Design review of the part built by this model. Coordinates are the model's own, in mm. A direction names the side the tool comes from. Round coordinates to 2 decimals unless told otherwise and drop trailing zeros. Order: outer loops, then holes, each group sorted by start corner. A loop starts at its lowest first (then second) coordinate and runs counter-clockwise, first axis right, second up.
from build123d import *

# Parameters (mm, degrees)
F1_DEPTH = 6.35
F2_W     = 6.35
F2_H     = 12.7
F3_DEPTH = 12.7


with BuildPart() as f1:
    # F0 (on Right) → F1 (new body, symmetric)
    with BuildSketch(Plane.YZ):
        Polygon((2.713958, 14.533968), (23.782384, 14.533968), (11.706621, 68.364052), (-39.854848, 68.364052), (-39.854848, 74.714052), (-52.554848, 74.714052), (-52.554848, 55.664052), (-1.754848, 55.664052), align=None)
    extrude(amount=F1_DEPTH, both=True)

    # F2 (on face) → F3 (join)
    with BuildSketch(Plane(origin=(0, 0, 14.533968), x_dir=(1, 0, 0), z_dir=(0, 0, -1))):
        with Locations((0, -14.143958)):
            Rectangle(F2_W, F2_H)
    extrude(amount=F3_DEPTH)


solid = f1.part
1) Take a section at D-D on x = -4.75. Give the boundary of the cut face in (y, z), plus the area to 3 significant figures.
Results:
outline: (-52.55, 55.66) - (-1.75, 55.66) - (2.71, 14.53) - (23.78, 14.53) - (11.71, 68.36) - (-39.85, 68.36) - (-39.85, 74.71) - (-52.55, 74.71) - close
area: 1,680 mm2
2) Take a section at A-A on x = 2. Give the boundary of the cut face in (y, z).
Results:
outline: (-52.55, 55.66) - (-1.75, 55.66) - (2.71, 14.53) - (7.79, 14.53) - (7.79, 1.83) - (20.49, 1.83) - (20.49, 14.53) - (23.78, 14.53) - (11.71, 68.36) - (-39.85, 68.36) - (-39.85, 74.71) - (-52.55, 74.71) - close
3) To check wall thickness, follow line 1 along Y through (x, z) = (1.25, 7.5); line 2 along Z through (x, y) = (-3.75, -15); line 3 along Z through (x, y) = (-4, 5). State the ranges of each line that lie inside material, in increasing order.
Results:
line 1: y = 7.79 to 20.49
line 2: z = 55.66 to 68.36
line 3: z = 14.53 to 68.36
4) Take a section at B-B on y = 10.5. Give the boundary of the cut face in (x, z) (3 decimals), plus the area to 3 significant figures.
Results:
outline: (-6.35, 14.534) - (-3.175, 14.534) - (-3.175, 1.834) - (3.175, 1.834) - (3.175, 14.534) - (6.35, 14.534) - (6.35, 68.364) - (-6.35, 68.364) - close
area: 764 mm2
5) Clearance check with flat-ended pins moving along their axes: P1, Ø6.5, axis at y = 15, z = 8.5, coming from the +X side (3 decimals); P2, Ø2, axis at x = -2, y = -20.5, coming from the +Z side; P3, Ø7, axis at x = 2, z = 73, coming from the +Y side. State where each tip first meets the part, or that it passes through.
Results:
P1: stops at x = 3.175
P2: stops at z = 68.36
P3: stops at y = -39.85
6) For faces 1 (the face through (-3.175, 14, 8)), 2 (the face through (0, 7.794, 8)), 3 (the face through (0, -39.855, 71)), list the 3-axis set-ups (+Z, -Z, +X, -X, +Y, -Y) from which the entire face can be reached by the end or side of a thin tool; tool diameter is ignored.
Results:
face 1: -Z, -X, +Y, -Y
face 2: -Z, +X, -X, -Y
face 3: +Z, +X, -X, +Y
7) Take a section at C-C on z = 23. Give the boundary of the cut face in (x, y).
Results:
outline: (-6.35, 1.79) - (6.35, 1.79) - (6.35, 21.88) - (-6.35, 21.88) - close
